Geometry check sheet. Reference: the model listing, model coordinates, mm. A direction names the side the tool comes from. Give positions to 0.01 mm unless a question says otherwise; leave off trailing zeros. Order: outer loops, then holes, each group sorted by start corner. A loop starts at its lowest first (then second) coordinate and runs counter-clockwise, first axis right, second up.
from build123d import *

# Parameters (mm, degrees)
F0_R           = 44
F1_DEPTH       = 68
F3_R           = 6
F4_DEPTH       = 10
F6_DEPTH       = 18
F8_ANGLE_BACK  = 10
F8_ANGLE       = 20
F12_ANGLE_BACK = 10
F12_ANGLE      = 20
F14_ANGLE_BACK = 10
F14_ANGLE      = 20


with BuildPart() as f1:
    # F0 (on Top) → F1 (new body)
    with BuildSketch(Plane.XY):
        Circle(F0_R)
        with BuildLine():
            ThreePointArc((-33.3407315568, 13.5792348554), (-29.4894735944, 20.6487517086), (-24.1635085752, 26.685667564))
            Line((-24.1635085752, 26.685667564), (-15.6760909215, 20.742713743))
            ThreePointArc((-15.6760909215, 20.742713743), (-12.0054639441, 23.0622816626), (-8, 24.7386337537))
            Line((-8, 24.7386337537), (-8, 35.0998575496))
            ThreePointArc((-8, 35.0998575496), (0, 36), (8, 35.0998575496))
            Line((8, 35.0998575496), (8, 24.7386337537))
            ThreePointArc((8, 24.7386337537), (12.0054639441, 23.0622816626), (15.6760909215, 20.742713743))
            Line((15.6760909215, 20.742713743), (24.1635085752, 26.685667564))
            ThreePointArc((24.1635085752, 26.685667564), (29.4894735944, 20.6487517086), (33.3407315568, 13.5792348554))
            Line((33.3407315568, 13.5792348554), (24.8533139031, 7.6362810343))
            ThreePointArc((24.8533139031, 7.6362810343), (0, -26), (-24.8533139031, 7.6362810343))
            Line((-24.8533139031, 7.6362810343), (-33.3407315568, 13.5792348554))
        make_face(mode=Mode.SUBTRACT)
    extrude(amount=F1_DEPTH)

    # F3 (on offset) → F4 (join)
    with BuildSketch(Plane.XY.offset(48)):
        with BuildLine():
            Line((-36.8781778292, -24), (-52.8015151298, -24))
            ThreePointArc((-52.8015151298, -24), (-38.6311115614, -43.2624227191), (-17.8938638331, -55.1707317073))
            ThreePointArc((-17.8938638331, -55.1707317073), (-9.0876412514, -63.6171726174), (-10.252187236, -75.7636022514))
            ThreePointArc((-10.252187236, -75.7636022514), (0, -94), (10.252187236, -75.7636022514))
            ThreePointArc((10.252187236, -75.7636022514), (9.0876412514, -63.6171726174), (17.8938638331, -55.1707317073))
            ThreePointArc((17.8938638331, -55.1707317073), (19.4267221495, -54.6498167108), (20.9444444444, -54.0863221796))
            ThreePointArc((20.9444444444, -54.0863221796), (39.8235273922, -42.1673649407), (52.8015151298, -24))
            Line((52.8015151298, -24), (36.8781778292, -24))
            ThreePointArc((36.8781778292, -24), (0, -44), (-36.8781778292, -24))
        make_face()
        with Locations((0, -82)):
            Circle(F3_R, mode=Mode.SUBTRACT)
        with BuildLine():
            Line((-52.8015151298, 24), (-36.8781778292, 24))
            ThreePointArc((-36.8781778292, 24), (0, 44), (36.8781778292, 24))
            Line((36.8781778292, 24), (52.8015151298, 24))
            ThreePointArc((52.8015151298, 24), (0, 58), (-52.8015151298, 24))
        make_face()
    extrude(amount=F4_DEPTH)

    # F5 (on Front) → F6 (join, symmetric)
    with BuildSketch(Plane.XZ):
        Polygon((56, 32), (39, 32), (39, 2.5551362713), align=None)
    extrude(amount=F6_DEPTH, both=True)

    # F7 (on Right) → F8 (revolve)
    with BuildSketch(Plane.YZ, mode=Mode.PRIVATE) as f8_sk:
        Polygon((-44, 58), (-44, 68), (-49, 58), align=None)
    revolve(f8_sk.sketch.rotate(Axis((0, 0, 36.8064753711), (0, 0, 1)), -F8_ANGLE_BACK), axis=Axis((0, 0, 36.8064753711), (0, 0, 1)), revolution_arc=F8_ANGLE)

    # F11 (on line) → F12 (revolve)
    with BuildSketch(Plane(origin=(0, 0, 0), x_dir=(-0.5735764364, 0.8191520443, 0), z_dir=(0.8191520443, 0.5735764364, 0)), mode=Mode.PRIVATE) as f12_sk:
        Polygon((-44, 58), (-44, 68), (-49, 58), align=None)
    revolve(f12_sk.sketch.rotate(Axis((0, 0, 36.8064753711), (0, 0, 1)), -F12_ANGLE_BACK), axis=Axis((0, 0, 36.8064753711), (0, 0, 1)), revolution_arc=F12_ANGLE)

    # F13 (on line) → F14 (revolve)
    with BuildSketch(Plane(origin=(0, 0, 0), x_dir=(0.5735764364, 0.8191520443, 0), z_dir=(0.8191520443, -0.5735764364, 0)), mode=Mode.PRIVATE) as f14_sk:
        Polygon((-49, 58), (-44, 58), (-44, 68), align=None)
    revolve(f14_sk.sketch.rotate(Axis((0, 0, 36.8064753711), (0, 0, 1)), -F14_ANGLE_BACK), axis=Axis((0, 0, 36.8064753711), (0, 0, 1)), revolution_arc=F14_ANGLE)


solid = f1.part
Item 1: Set-up check for faces 1 (the flat face through (-19.979, 23.756, 33.524)), 2 (the flat face through (46, -18, 22)), 3 (the flat face through (19.2, -41.17, 60.85)): record each of +Z, -Z, +X, -X, +Y, -Y from which the full face is reachable in a straight line by a thin tool's end or side.
Reported:
face 1: +Z, -Z
face 2: +Z, -Z, +X, -Y
face 3: +Z, -Y
Item 2: Sectioned sample at A-A (y = -82). Enter the section's corners in (x, z).
Reported:
outline: (-12, 48) - (-6, 48) - (-6, 58) - (-12, 58) - close; (6, 48) - (12, 48) - (12, 58) - (6, 58) - close
Item 3: Sectioned sample at D-D (y = -3). Enter the section's corners in (x, z), and give its area (3 significant figures).
Reported:
outline: (-43.9, 0) - (-25.83, 0) - (-25.83, 68) - (-43.9, 68) - close; (25.83, 0) - (43.9, 0) - (43.9, 11.04) - (56, 32) - (43.9, 32) - (43.9, 68) - (25.83, 68) - close
area: 2,580 mm2
Item 4: Sectioned sample at C-C (z = 38). Enter the section's corners in (x, y), and give its area (3 significant figures).
Reported:
outline: circle Ø88 at (0, 0); hole (-33.34, 13.58) - (-24.85, 7.64) arc R26 ccw (long way) to (24.85, 7.64) - (33.34, 13.58) arc R36 ccw to (24.16, 26.69) - (15.68, 20.74) arc R26 ccw to (8, 24.74) - (8, 35.1) arc R36 ccw to (-8, 35.1) - (-8, 24.74) arc R26 ccw to (-15.68, 20.74) - (-24.16, 26.69) arc R36 ccw to start
area: 3,470 mm2
Item 5: Draft check along Y on faces 4 (the conical face through (26.6, -38.2, 62.9)), 5 (the flat face through (-1, 45, 58)), 6 (the cylindrical face through (0.929, 57.993, 52.93)), 7 (the flat face through (45, -24, 53)). Enter one of: released by +Y, released by -Y, zero draft, split by the parting line, or undercut.
Reported:
face 4: released by -Y
face 5: zero draft
face 6: released by +Y
face 7: undercut
Item 6: Scan lines: L1, parallel to Y at x = 0, z = 53; L2, parallel to Y at x = 0, z = 34; L3, parallel to X at y = 21, z = 34.5. Record each from-to range of solid material in increasing order.
Reported:
L1: y = -94 to -88, -76 to -26, 36 to 58
L2: y = -44 to -26, 36 to 44
L3: x = -38.67 to -29.24, -16.04 to -15.33, 15.33 to 16.04, 29.24 to 38.67
Item 7: Gauge pin test, flat ends, axial feed: pin 1 (14 mm diameter, centred on x = 0, y = -82, fed in from -Z); pin 2 (5 mm diameter, centred on x = 46.5, z = 53, fed in from +Y); pin 3 (1 mm diameter, centred on y = 33, z = 20.5, fed in from +X). Record the tip position at first contact, or that the pin passes through.
Reported:
pin 1: stops at z = 48
pin 2: stops at y = 37.79
pin 3: stops at x = 29.66
Item 8: Sectioned sample at B-B (x = 0). Enter the section's corners in (y, z), and give its area (3 significant figures).
Reported:
outline: (-94, 48) - (-88, 48) - (-88, 58) - (-94, 58) - close; (-76, 48) - (-44, 48) - (-44, 0) - (-26, 0) - (-26, 68) - (-44, 68) - (-49, 58) - (-76, 58) - close; (36, 0) - (44, 0) - (44, 48) - (58, 48) - (58, 58) - (44, 58) - (44, 68) - (36, 68) - close
area: 2,310 mm2
